Part model, mm, in its own coordinate system. A direction names the side the tool comes from. Give positions to 0.01 mm unless a question says otherwise; leave off trailing zeros. Write each loop counter-clockwise with the first axis right and the second up, starting at its lowest first coordinate (ties: lowest second). Pieces come first, ordered by that corner, then holes. Notation, with made-up numbers: M -39.75,24 L -9.75,24 A23 ccw -9.75,57 Z; hole C 47.5,1 d3. An arc over 180 degrees is marked long. Answer as CSV lines item,"result". Start each with the question number.
1) Pin check, flat tips, straight feed: pin 1 Ø8 at (x, z) = (2.5, 1.5) entering from -Y; pin 2 Ø1 at (x, z) = (1.5, -3) entering from -Y. Stop position of each tip, or through.
2) Wall check: line 1 along Z through (x, y) = (-0.25, 1.5); line 2 along Y through (x, z) = (0, 4.25); line 3 along X through (y, z) = (19.75, 9). Give the ranges that are in metal, low to high. Write a range as from..to.
3) Slice it at B-B, the plane x = 0. Give the cut face in (y, z).
4) Slice it at C-C, the plane z = 0. Give the cut face in (x, y), plus the area to 3 significant figures.
5) Tool access for faces 1 (the cylindrical face through (-1.08, 3.94, -4.88)), 2 (the flat face through (0, 11, -10)): list every direction of +Z, -Z, +X, -X, +Y, -Y with a clear straight run to the whole face (end or side of a thin tool).
6) Slice it at A-A, the plane y = 20. Give the cut face in (x, z), plus the area to 3 significant figures.
7) Mould opens along X. For faces 3 (the flat face through (-2, 0, -5)), 4 (the flat face through (10, 15, 0)), 5 (the flat face through (-10, 15, 0)), 6 (the flat face through (0, 8, 0)) say: pulls with the +X half, pulls with the -X half, needs draft (parallel to the pull), parting line crosses it, or undercut.
8) Slice it at D-D, the plane y = 3.75. Give the cut face in (x, z).
```python
from build123d import *

# Parameters (mm, degrees)
SKETCH1_W           = 20
SKETCH1_H           = 20
BOSS_EXTRUDE2_DEPTH = 30
CUT_EXTRUDE1_REACH  = 22
SKETCH2_R           = 6
SKETCH3_R           = 5
CUT_EXTRUDE2_DEPTH  = 8


with BuildPart() as part:
    # Sketch1 → Boss-Extrude2 (new body)
    with BuildSketch(Plane(origin=(0, 0, 0), x_dir=(1, 0, 0), z_dir=(0, 1, 0))):
        Rectangle(SKETCH1_W, SKETCH1_H)
    extrude(amount=BOSS_EXTRUDE2_DEPTH)

    # Sketch2 → Cut-Extrude1 (cut, up to next)
    with BuildSketch(Plane.XY.offset(10), mode=Mode.PRIVATE) as cut_extrude1_sk1:
        with Locations((0, 20)):
            Circle(SKETCH2_R)
    cut_extrude1_tool1 = extrude(cut_extrude1_sk1.sketch, amount=-CUT_EXTRUDE1_REACH, mode=Mode.PRIVATE) & part.part
    add(cut_extrude1_tool1.solids().sort_by_distance((0, 20, 10))[0], mode=Mode.SUBTRACT)

    # Sketch3 → Cut-Extrude2 (cut)
    with BuildSketch(Plane.XZ):
        Circle(SKETCH3_R)
    extrude(amount=-CUT_EXTRUDE2_DEPTH, mode=Mode.SUBTRACT)


solid = part.part
```
Found:
1,pin 1,"y = 0"
1,pin 2,"y = 8"
2,line 1,"-10..-4.99, 4.99..10"
2,line 2,"8..14, 26..30"
2,line 3,"-10..-5.99, 5.99..10"
3,outline,"M 0,-10 L 14,-10 L 14,10 L 0,10 L 0,5 L 8,5 L 8,-5 L 0,-5 Z; M 26,-10 L 30,-10 L 30,10 L 26,10 Z"
4,outline,"M -10,0 L -5,0 L -5,8 L 5,8 L 5,0 L 10,0 L 10,30 L -10,30 Z; hole C 0,20 d12"
4,area,"407 mm²"
5,face 1,"-Y"
5,face 2,"-Z, +X, -X, +Y, -Y"
6,outline,"M -10,-10 L -6,-10 L -6,10 L -10,10 Z; M 6,-10 L 10,-10 L 10,10 L 6,10 Z"
6,area,"160 mm²"
7,face 3,"needs draft"
7,face 4,"pulls with the +X half"
7,face 5,"pulls with the -X half"
7,face 6,"undercut"
8,outline,"M -10,-10 L 10,-10 L 10,10 L -10,10 Z; hole C 0,0 d10"
